Input: part model. Units: mm. Frame: model coordinates. A direction names the side the tool comes from. Give positions to 0.01 mm unless a question says otherwise; leave off trailing zeros. Write each loop counter-clockwise with the first axis right and the second up, starting at its lowest first coordinate (ties: lowest second). Pieces come first, ordered by that corner, then holes. Notation, with made-up numbers: (85, 51.5) -> (129, 51.5) arc R27 cw to (129, 83.5) -> close; hole circle Ø4 at (65.25, -1). An arc over 180 degrees is marked (long way). Return JSON: item names as keys, results as strings. Group by question number.
Item 1: Section A-A, the plane y = 6.5. Return loops of the section in (x, z), then the cut area to 3 significant figures.
Item 2: Mould query, pull axis X, two halves, no side actions, for faces 5 (the face through (15, 40, -5)), 6 (the face through (-9.2, 2, -5)), 7 (the face through (7, 34.81, -5)), 8 (the face through (17.8, 45, -5)). Classes: released by +X, released by -X, zero draft, split by the parting line, or undercut.
Item 3: Section D-D, the plane x = 22. Return loops of the section in (y, z).
Item 4: Pin query (flat end, axial travel): P1, Ø5, axis at y = 14.5, z = -8, coming from the +X side; P2, Ø2, axis at x = 0, z = -2.5, coming from the +Y side; P3, Ø3.5, axis at x = -6, z = -5, coming from the +Y side. Return the tip coordinate at first contact, or that it passes through.
Item 5: Set-up query: faces 1 (the face through (-7.578, 1.965, -7.784)), 2 (the face through (1.154, 44.232, -4.93)), 3 (the face through (-5.1, 3, -1.6)), 4 (the face through (-7.4, 0, -3.8)). Return all of +Z, -Z, +X, -X, +Y, -Y with unobstructed straight access to the full face (end or side cutting, diameter ignored); none if empty.
Item 6: Section C-C, the plane z = -7.5. Return loops of the section in (x, y), then the cut area to 3 significant figures.
Item 7: Section B-B, the plane x = 7.5. Return loops of the section in (y, z), then the cut area to 3 significant figures.
Item 8: Line query: line 1 (X direction, y = 12, z = -7); line 2 (X direction, y = 0.2, z = -5); line 3 (Y direction, x = 6, z = -4.5). Output: solid intervals per line, ascending. Write a range as [from, to].
from build123d import *

# Parameters (mm, degrees)
BOSS_EXTRUDE1_DEPTH = 10
BOSS_EXTRUDE2_REACH = 65.68
SKETCH3_R           = 1.6
CUT_EXTRUDE1_DEPTH  = 2.1
SKETCH3_2_R         = 1.6
CUT_EXTRUDE2_DEPTH  = 55.597829326
SKETCH4_R           = 1.6
CUT_EXTRUDE3_DEPTH  = 2.1
SKETCH4_4_R         = 1.6
CUT_EXTRUDE4_DEPTH  = 55.958571782


with BuildPart() as part:
    # Sketch1 → Boss-Extrude1 (new body)
    with BuildSketch(Plane.XY):
        Polygon((-12, 0), (0, 0), (0, 34.81), (15, 34.81), (15, 44.81), (30, 44.81), (30, 46.81), (-12, 46.81), align=None)
        Polygon((12, 36.81), (-2, 36.81), (-2, 3), (-10, 3), (-10, 44.81), (12, 44.81), align=None, mode=Mode.SUBTRACT)
    extrude(amount=-BOSS_EXTRUDE1_DEPTH)

    # Boss-Extrude2: up to this face of the body (flat: up to its plane)
    boss_extrude2_end = Plane(part.part.faces().sort_by_distance((-12, 23.405, -5))[0])
    # Sketch2 → Boss-Extrude2 (add, up to the picked face)
    with BuildSketch(Plane(origin=(30, 0, 0), x_dir=(0, 0, -1), z_dir=(1, 0, 0)), mode=Mode.PRIVATE) as boss_extrude2_sk1:
        Polygon((10, 47.949356083), (0, 46.81), (10, 46.81), align=None)
    boss_extrude2_tool1 = split(extrude(boss_extrude2_sk1.sketch, amount=-BOSS_EXTRUDE2_REACH, mode=Mode.PRIVATE), bisect_by=boss_extrude2_end, keep=Keep.BOTH, mode=Mode.PRIVATE)
    # Sketch2 → Boss-Extrude2 (add, up to the picked face)
    with BuildSketch(Plane(origin=(30, 0, 0), x_dir=(0, 0, -1), z_dir=(1, 0, 0)), mode=Mode.PRIVATE) as boss_extrude2_sk2:
        Polygon((10, 44.81), (0, 44.81), (0, 43.670643917), align=None)
    boss_extrude2_tool2 = split(extrude(boss_extrude2_sk2.sketch, amount=-BOSS_EXTRUDE2_REACH, mode=Mode.PRIVATE), bisect_by=boss_extrude2_end, keep=Keep.BOTH, mode=Mode.PRIVATE)
    add(boss_extrude2_tool1.solids().sort_by(Axis((30, 47.189785, -6.666667), (-1, 0, 0)))[0])
    add(boss_extrude2_tool2.solids().sort_by(Axis((30, 44.430215, -3.333333), (-1, 0, 0)))[0])

    # Sketch3 → Cut-Extrude1 (cut)
    with BuildSketch(Plane(origin=(0, 43.11100603, 4.911878697), x_dir=(1, 0, 0), z_dir=(0, -0.9935718556765883, -0.11320321376790003))):
        Polygon((24.2, -8.128485041), (21, -6.280964179), (17.8, -8.128485041), (17.8, -11.823526764), (21, -13.671047625), (24.2, -11.823526764), align=None)
        with Locations(Location((21, -9.976005902, 0), (0, 0, 270))):
            Circle(SKETCH3_R, mode=Mode.SUBTRACT)
    extrude(amount=-CUT_EXTRUDE1_DEPTH, mode=Mode.SUBTRACT)

    # Sketch3<2> → Cut-Extrude2 (cut, through all)
    with BuildSketch(Plane(origin=(0, 43.11100603, 4.911878697), x_dir=(1, 0, 0), z_dir=(0, -0.9935718556765883, -0.11320321376790003))):
        with Locations(Location((21, -9.976005902, 0), (0, 0, 270))):
            Circle(SKETCH3_2_R)
    extrude(amount=-CUT_EXTRUDE2_DEPTH, mode=Mode.SUBTRACT)

    # Sketch4 → Cut-Extrude3 (cut)
    with BuildSketch(Plane(origin=(0, 3, 0), x_dir=(1, 0, 0), z_dir=(0, 1, 0))):
        Polygon((-2.8, 3.152479139), (-2.8, 6.847520861), (-6, 8.695041723), (-9.2, 6.847520861), (-9.2, 3.152479139), (-6, 1.304958277), align=None)
        with Locations(Location((-6, 5, 0), (0, 0, 270))):
            Circle(SKETCH4_R, mode=Mode.SUBTRACT)
    extrude(amount=-CUT_EXTRUDE3_DEPTH, mode=Mode.SUBTRACT)

    # Sketch4<4> → Cut-Extrude4 (cut, through all)
    with BuildSketch(Plane(origin=(0, 3, 0), x_dir=(1, 0, 0), z_dir=(0, 1, 0))):
        with Locations(Location((-6, 5, 0), (0, 0, 270))):
            Circle(SKETCH4_4_R)
    extrude(amount=-CUT_EXTRUDE4_DEPTH, mode=Mode.SUBTRACT)


solid = part.part
Answer below:
{
 "1": {"outline": "(-12, -10) -> (-10, -10) -> (-10, 0) -> (-12, 0) -> close; (-2, -10) -> (0, -10) -> (0, 0) -> (-2, 0) -> close", "area": "40.0 mm2"},
 "2": {"face 5": "released by +X", "face 6": "undercut", "face 7": "zero draft", "face 8": "undercut"},
 "3": {"outline": "(43.67, 0) -> (43.89, -1.9) -> (45.97, -1.66) -> (46.19, -3.52) -> (47.2, -3.41) -> (46.81, 0) -> close; (44.59, -8.1) -> (44.81, -10) -> (47.95, -10) -> (47.48, -5.89) -> (46.47, -6) -> (46.68, -7.86) -> close"},
 "4": {"P1": "stops at x = 0", "P2": "stops at y = 47.21", "P3": "stops at y = 47.58"},
 "5": {"face 1": "none", "face 2": "-Z", "face 3": "+Z, -Z", "face 4": "+Z, -Z, +X, -X, -Y"},
 "6": {"outline": "(-12, 0) -> (0, 0) -> (0, 34.81) -> (15, 34.81) -> (15, 44.53) -> (18.96, 44.53) -> (19.37, 46.64) -> (22.63, 46.64) -> (23.04, 44.53) -> (30, 44.53) -> (30, 47.66) -> (-12, 47.66) -> close; hole (-10, 3) -> (-8.07, 3) -> (-8.07, 0.9) -> (-3.93, 0.9) -> (-3.93, 3) -> (-2, 3) -> (-2, 36.81) -> (12, 36.81) -> (12, 44.53) -> (-10, 44.53) -> close", "area": "355 mm2"},
 "7": {"outline": "(34.81, -10) -> (36.81, -10) -> (36.81, 0) -> (34.81, 0) -> close; (43.67, 0) -> (44.81, -10) -> (47.95, -10) -> (46.81, 0) -> close", "area": "51.4 mm2"},
 "8": {"line 1": "x = [-12, -10], [-2, 0]", "line 2": "x = [-12, -7.6], [-4.4, 0]", "line 3": "y = [34.81, 36.81], [44.18, 47.32]"}
}
